```python
from build123d import *

# Parameters (mm, degrees)
F0_R     = 97
F1_DEPTH = 112.5


with BuildPart() as f1:
    # F0 (on Top) → F1 (new body, symmetric)
    with BuildSketch(Plane.XY):
        with BuildLine():
            ThreePointArc((138.247517, -22.082214), (139.561191, -11.075822), (140, 0))
            ThreePointArc((140, 0), (115.325626, 79.372539), (50, 130.766968))
            ThreePointArc((50, 130.766968), (0, 140), (-50, 130.766968))
            ThreePointArc((-50, 130.766968), (-121.243557, 70), (-138.247517, -22.082214))
            ThreePointArc((-138.247517, -22.082214), (-121.243557, -70), (-88.247517, -108.684754))
            ThreePointArc((-88.247517, -108.684754), (0, -140), (88.247517, -108.684754))
            ThreePointArc((88.247517, -108.684754), (121.243557, -70), (138.247517, -22.082214))
        make_face()
        Circle(F0_R, mode=Mode.SUBTRACT)
    extrude(amount=F1_DEPTH, both=True)


solid = f1.part
```
Source: CAD feature listing. Evaluate the final solid. Frame: model axes, mm. Give positions to 0.01 mm unless a question says otherwise; leave off trailing zeros. Loops run counter-clockwise (first coordinate to the right, second up) from the corner with the lowest first, then second, coordinate; pieces in that order, holes last. Notation, with made-up numbers: (32.25, -14.5) - (79.25, -14.5) arc R6 cw to (79.25, -7.5) - close; hole circle Ø6 at (52.5, -23). An arc over 180 degrees is marked (long way). Use CSV: the item, a comma, the result in double quotes. Start each with the question number.
1. Pin query (flat end, axial travel): pin 1 (5 mm diameter, centred on x = 37, z = 26.5, fed in from -Y); pin 2 (8 mm diameter, centred on y = 84.5, z = -11.5, fed in from -X); pin 3 (5 mm diameter, centred on x = 98, z = 27.5, fed in from +Y). Return the tip coordinate at first contact, or that it passes through.
2. Ray query, L1, parallel to Y at x = 0, z = 45; L2, parallel to X at y = 66.5, z = -52; L3, parallel to X at y = 21, z = -96.5. Return the intervals inside material, ascending.
3. Section B-B (z = 23.5). Output: boundary loops of the cut face in (x, y), then the cut area to 3 significant figures.
4. Draft query along Y for faces 1 (the cylindrical face through (139.55, -11.23, 1.58)), 2 (the cylindrical face through (44.76, -86.056, -1.575)), 3 (the flat face through (-33.1, -91.4, 112.5)). Return one class per face: +Y half, -Y half, draft (parallel to the pull), parting line (faces both ways), or undercut.
5. Section A-A (x = 0). Output: boundary loops of the cut face in (y, z).
6. Section D-D (y = 104). Output: boundary loops of the cut face in (x, z).
7. Section C-C (y = -83.5). Output: boundary loops of the cut face in (x, z).
Response:
1,pin 1,"y = -135.68"
1,pin 2,"x = -114.54"
1,pin 3,"y = 102.37"
2,L1,"-140 to -97, 97 to 140"
2,L2,"-123.2 to -70.62, 70.62 to 123.2"
2,L3,"-138.42 to -94.7, 94.7 to 138.42"
3,outline,"(-88.25, -108.68) arc R140 ccw to (88.25, -108.68) arc R140 ccw to (138.25, -22.08) arc R140 ccw to (140, 0) arc R140 ccw to (50, 130.77) arc R140 ccw to (-50, 130.77) arc R140 ccw to start; hole circle Ø194 at (0, 0)"
3,area,"32,000 mm²"
4,face 1,"-Y half"
4,face 2,"undercut"
4,face 3,"draft"
5,outline,"(-140, -112.5) - (-97, -112.5) - (-97, 112.5) - (-140, 112.5) - close; (97, -112.5) - (140, -112.5) - (140, 112.5) - (97, 112.5) - close"
6,outline,"(-93.72, -112.5) - (93.72, -112.5) - (93.72, 112.5) - (-93.72, 112.5) - close"
7,outline,"(-112.37, -112.5) - (-49.36, -112.5) - (-49.36, 112.5) - (-112.37, 112.5) - close; (49.36, -112.5) - (112.37, -112.5) - (112.37, 112.5) - (49.36, 112.5) - close"
